Work out the finished part from the listing and answer in its coordinate system (mm). Give positions to 0.01 mm unless a question says otherwise; leave off trailing zeros. Write each loop counter-clockwise with the first axis right and the second up, starting at its lowest first coordinate (ties: lowest second). Pieces come first, ordered by that corner, then holes.
1) Find section A-A (z = 28). Determine the outline of the cut face in (x, y) (3 decimals).
2) Find section C-C (y = -9). Determine the outline of the cut face in (x, z), plus the area to 3 significant figures.
3) Find section B-B (z = -7). Determine the outline of the cut face in (x, y) (3 decimals).
4) Straight lines are drawn through the part: probe 1 along Y at (x, z) = (8.5, 29) (3 decimals); probe 2 along Y at (x, z) = (7, 8) (3 decimals); probe 3 along Z at (x, y) = (2.25, 4.5). For each, find the intervals that lie inside material, in ascending order.
5) Given pin 1 Ø3 at (x, y) = (4, -92.5) entering from -Z (3 decimals); pin 2 Ø1 at (y, z) = (9.5, 2.5) entering from -X; pin 3 Ø1.5 at (x, y) = (2.5, 58.5) entering from -Z; pin 4 Ø5 at (x, z) = (5.5, -31) entering from +Y (3 decimals), each flat-ended and moving along its own axis, determine where each tip first touches the part or whether it passes through.
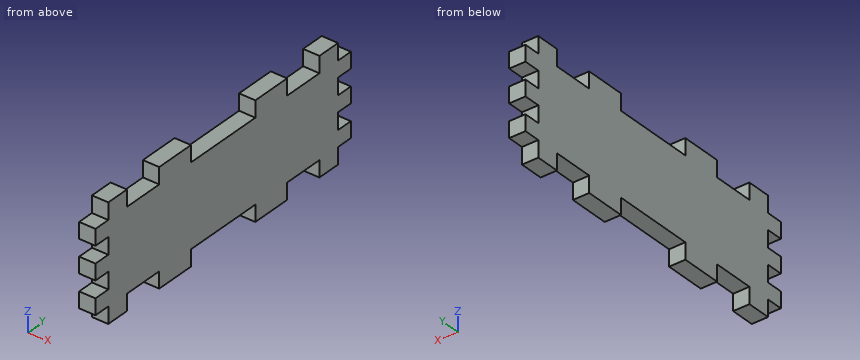
```python
from build123d import *

# Parameters (mm, degrees)
F1_DEPTH = 10


with BuildPart() as f1:
    # F0 (on Right) → F1 (new body)
    with BuildSketch(Plane.YZ):
        Polygon((-99.625, -24.875), (-89.625, -24.875), (-89.625, -35), (-75.125, -35), (-75.125, -25), (-49.875, -25), (-49.875, -35), (-25.125, -35), (-25.125, -25), (0, -25), (25.125, -25), (25.125, -35), (49.875, -35), (49.875, -25), (75.125, -25), (75.125, -35), (89.625, -35), (89.625, -24.875), (99.625, -24.875), (99.625, -15.125), (89.625, -15.125), (89.625, -4.875), (99.625, -4.875), (99.625, 0), (99.625, 4.875), (89.625, 4.875), (89.625, 15.125), (99.625, 15.125), (99.625, 24.875), (89.625, 24.875), (89.625, 35), (75.125, 35), (75.125, 25), (49.875, 25), (49.875, 35), (25.125, 35), (25.125, 25), (0, 25), (-25.125, 25), (-25.125, 35), (-49.875, 35), (-49.875, 25), (-75.125, 25), (-75.125, 35), (-89.625, 35), (-89.625, 24.875), (-99.625, 24.875), (-99.625, 15.125), (-89.625, 15.125), (-89.625, 4.875), (-99.625, 4.875), (-99.625, 0), (-99.625, -4.875), (-89.625, -4.875), (-89.625, -15.125), (-99.625, -15.125), align=None)
    extrude(amount=F1_DEPTH)


solid = f1.part
```
Results:
1. outline: (0, -89.625) - (10, -89.625) - (10, -75.125) - (0, -75.125) - close; (0, -49.875) - (10, -49.875) - (10, -25.125) - (0, -25.125) - close; (0, 25.125) - (10, 25.125) - (10, 49.875) - (0, 49.875) - close; (0, 75.125) - (10, 75.125) - (10, 89.625) - (0, 89.625) - close
2. outline: (0, -25) - (10, -25) - (10, 25) - (0, 25) - close
2. area: 500 mm2
3. outline: (0, -89.625) - (10, -89.625) - (10, 89.625) - (0, 89.625) - close
4. probe 1: y = -89.625 to -75.125, -49.875 to -25.125, 25.125 to 49.875, 75.125 to 89.625
4. probe 2: y = -89.625 to 89.625
4. probe 3: z = -25 to 25
5. pin 1: stops at z = -24.875
5. pin 2: stops at x = 0
5. pin 3: stops at z = -25
5. pin 4: stops at y = 89.625
